For this review, take the finished solid that the model builds, in its own axes (mm). A direction names the side the tool comes from. Coordinates: 2 decimals unless noted, no trailing zeros. Write each loop counter-clockwise with the first axis right and the second up, starting at its lowest first coordinate (ties: lowest second). Pieces come first, ordered by that corner, then holes.
Autodesk Inventor part; units mm, degrees
ref_plane "YZ Plane" through (0, 0, 0) normal (1, 0, 0) x (0, 1, 0)
ref_plane "XZ Plane" through (0, 0, 0) normal (0, 1, 0) x (-1, 0, 0)
ref_plane "XY Plane" through (0, 0, 0) normal (0, 0, 1) x (1, 0, 0)
ref_plane "Plano de trabajo1" through (0, 0, 0) normal (0, 0, 1) x (1, 0, 0)
sketch "Boceto1" plane through (0, 0, 0) normal (0, 0, 1) x (1, 0, 0)
  circle A0 centre (10.9923, -7.35) radius 1.2028
  circle A1 centre (3.6423, 0) radius 1.2028
  circle A2 centre (18.3423, 0) radius 1.2028
  circle A3 centre (10.9923, 7.35) radius 1.2028
  circle A4 centre (10.9923, 0) radius 10.9823
  line L0 (10.9923, -10.9823) -> (-139.0077, -10.9823)
  line L1 (10.9923, 10.9823) -> (-139.0077, 10.9823)
  line L2 (-139.0077, 10.9823) -> (-139.0077, -10.9823)
  point P0 (0, 0)
  dimension "d0" = 150
  dimension "d1" = 150
extrude "Extrusión1" add sketch "Boceto1" along normal blind 3
sketch "Boceto2" plane through (0, 0, 3) normal (0, 0, 1) x (1, 0, 0)
  arc A0 (-129.1978, -5.6745) -> (-132.1454, -8.5217) centre (-128.1245, -9.7351) ccw
  circle A1 centre (-128.1245, 8.4649) radius 0.85 construction
  circle A2 centre (-128.1245, -9.7351) radius 0.7049 construction
  line L0 (-139.0305, -11.0697) -> (-267.2186, 10.8953)
  line L1 (-267.2186, -11.0694) -> (-117.2186, -11.0694)
  line L2 (-139.0305, 10.8953) -> (-139.0305, -11.0694)
  line L3 (-117.2186, 10.8953) -> (-267.2186, 10.8953)
  line L4 (-128.1245, -11.0697) -> (-128.1245, -0.0872)
  line L5 (-128.1245, -0.0872) -> (-128.1245, 9.0128)
  line L6 (-128.1245, -0.0872) -> (-128.1245, -9.1872)
  circle A3 centre (-128.1245, -9.1872) radius 0.85
  circle A4 centre (-128.1245, 9.0128) radius 0.85
  circle A5 centre (-128.1245, -9.1872) radius 1.8825
  circle A6 centre (-128.1245, 9.0128) radius 1.8821
  circle A7 centre (-128.1245, 9.0128) radius 0.85
  circle A8 centre (-128.1245, -9.1872) radius 0.85
  line L7 (-128.1245, 10.8953) -> (-139.0305, 10.8953)
  line L8 (-139.0077, 10.9823) -> (-139.0077, -10.9823)
  line L9 (-139.0077, -10.9823) -> (-139.0077, 10.9823)
  line L10 (-139.0077, 10.9823) -> (-139.0077, -10.9823)
  point P0 (0, 0)
  dimension "d4" = 10.9825
  dimension "d5" = 9.1
  dimension "d6" = 9.1
  dimension "d7" = 1.7
  dimension "d8" = 1.7
extrude "Extrusión2" cut sketch "Boceto2" against normal blind 3 contours A3 L4 | L4 A3 | A4
sketch "Boceto3" plane through (0, 0, 3) normal (0, 0, 1) x (1, 0, 0)
  circle A0 centre (-128.1245, -9.1872) radius 0.85
  circle A1 centre (-128.1245, 9.0128) radius 0.85
  line L0 (10.9923, 10.9823) -> (-139.0077, 10.9823)
  line L1 (-139.0077, 10.9823) -> (-139.0077, -10.9823)
  line L2 (-139.0077, -10.9823) -> (10.9923, -10.9823)
  arc A2 (10.9923, -10.9823) -> (10.9923, 10.9823) centre (10.9923, 0) ccw
  circle A3 centre (10.9923, -7.35) radius 1.2028
  circle A4 centre (3.6423, 0) radius 1.2028
  circle A5 centre (18.3423, 0) radius 1.2028
  circle A6 centre (10.9923, 7.35) radius 1.2028
  line L3 (-130.1442, 5.5225) -> (-129.5361, 14.2169)
  circle A7 centre (-128.1245, -9.1872) radius 1.7951
  circle A8 centre (-128.1245, 9.0128) radius 1.9695
  line L4 (-128.1245, -7.3921) -> (-128.1245, 7.0432)
  line L5 (-128.1245, -10.9823) -> (-128.1245, -18.0451)
  line L6 (-128.1245, -18.0451) -> (-142.6221, -18.554)
  line L7 (-142.6221, -18.554) -> (-141.7315, 12.8288)
  line L8 (-141.7315, 12.8288) -> (-128.1245, 12.4426)
  line L9 (-128.1245, 12.4426) -> (-128.1245, 10.9823)
  point P0 (0, 0)
extrude "Extrusión3" cut sketch "Boceto3" against normal blind 3 contours A8 L3 L0 | L3 A8 L4 A7 L2 L1 L0
sketch "Boceto4" plane through (0, 0, 0) normal (0, 0, -1) x (-1, 0, 0)
  arc A0 (128.1245, 7.0432) -> (128.1245, 10.9823) centre (128.1245, 9.0128) ccw
  line L0 (-10.9923, 10.9823) -> (128.1245, 10.9823)
  arc A1 (-10.9923, 10.9823) -> (-10.9923, -10.9823) centre (-10.9923, 0) ccw
  line L1 (128.1245, -10.9823) -> (-10.9923, -10.9823)
  arc A2 (128.1245, -10.9823) -> (128.1245, -7.3921) centre (128.1245, -9.1872) ccw
  line L2 (128.1245, -7.3921) -> (128.1245, 7.0432)
  circle A3 centre (128.1245, -9.1872) radius 0.85
  circle A4 centre (128.1245, 9.0128) radius 0.85
  circle A5 centre (-10.9923, -7.35) radius 1.2028
  circle A6 centre (-3.6423, 0) radius 1.2028
  circle A7 centre (-18.3423, 0) radius 1.2028
  circle A8 centre (-10.9923, 7.35) radius 1.2028
  line L3 (108.1857, 10.9823) -> (108.1857, -10.9823)
  point P0 (0, 0)
extrude "Extrusión4" add sketch "Boceto4" along normal blind 12 contours L2 A2 L1 L3 L0 A0
sketch "Boceto5" plane through (0, 0, 3) normal (0, 0, 1) x (1, 0, 0)
  line L0 (-108.1857, -10.9823) -> (-108.1857, 10.9823)
  circle A0 centre (10.9923, 7.35) radius 1.2028
  circle A1 centre (18.3423, 0) radius 1.2028
  circle A2 centre (3.6423, 0) radius 1.2028
  circle A3 centre (10.9923, -7.35) radius 1.2028
  arc A4 (-128.1245, 10.9823) -> (-128.1245, 7.0432) centre (-128.1245, 9.0128) ccw
  line L1 (-128.1245, 7.0432) -> (-128.1245, -7.3921)
  arc A5 (-128.1245, -7.3921) -> (-128.1245, -10.9823) centre (-128.1245, -9.1872) ccw
  line L2 (-128.1245, -10.9823) -> (10.9923, -10.9823)
  arc A6 (10.9923, -10.9823) -> (10.9923, 10.9823) centre (10.9923, 0) ccw
  line L3 (10.9923, 10.9823) -> (-128.1245, 10.9823)
  circle A7 centre (-128.1245, 9.0128) radius 0.85
  circle A8 centre (-128.1245, -9.1872) radius 0.85
  line L4 (-108.1857, 10.9823) -> (-111.1857, 10.9823)
  line L5 (-111.1857, 10.9823) -> (-111.1857, -10.9823)
  line L6 (-111.1857, -10.9823) -> (-108.1857, -10.9823)
  line L7 (-108.1857, -10.9823) -> (-108.1857, 10.9823)
  line L8 (10.9923, 10.9823) -> (-128.1245, 10.9823)
  line L9 (-122.3999, 10.9823) -> (-122.3999, -10.9823)
  point P0 (0, 0)
  dimension "d15" = 3
extrude "Extrusión5" cut sketch "Boceto5" against normal blind 13 contours L2 A5 L1 A4 L3 L9
chamfer "Chaflán1" distance 12 angle 45 1 edges at (-122.3999, 0, 3)
chamfer "Chaflán2" distance 12 angle 45 1 edges at (-108.1857, 0, -12)
sketch "Boceto6" plane through (0, 0, -12) normal (0, 0, -1) x (-1, 0, 0)
  line L0 (126.0445, -11.1372) -> (126.0445, 10.9228)
  line L1 (120.1857, -10.9823) -> (120.1857, 10.9823)
  line L2 (120.1857, -10.9823) -> (128.1245, -10.9823)
  line L3 (120.1857, 10.9823) -> (122.6857, 10.9823)
  line L4 (122.6857, 10.9823) -> (122.6857, -10.9823)
  line L5 (122.6857, -10.9823) -> (120.1857, -10.9823)
  line L6 (120.1857, -10.9823) -> (120.1857, 10.9823)
  point P0 (0, 0)
  dimension "d24" = 2.5
extrude "Extrusión6" add sketch "Boceto6" along normal blind 20
sketch "Boceto7" plane through (-128.1245, -10.9823, -10) normal (0, -1, 0) x (1, 0, 0)
  line L0 (19.9388, 10) -> (7.9388, -2)
  line L1 (19.9388, 10) -> (139.1168, 10)
  line L2 (139.1168, 10) -> (139.1168, 13)
  line L3 (17.7246, 13) -> (139.1168, 13)
  line L4 (5.7246, 1) -> (17.7246, 13)
  line L5 (5.7246, 1) -> (5.7246, 0)
  line L6 (5.7246, 0) -> (0, 0)
  line L7 (0, 0) -> (0, -2)
  line L8 (5.4388, -2) -> (0, -2)
  line L9 (5.4388, -2) -> (5.4388, -22)
  line L10 (7.9388, -22) -> (5.4388, -22)
  line L11 (7.9388, -2) -> (7.9388, -22)
  line L12 (7.9388, -2) -> (7.9388, -22)
  line L13 (5.4388, -22) -> (7.9388, -22)
  line L14 (7.9388, -22) -> (7.9388, -4)
  line L15 (7.9388, -4) -> (5.4388, -4)
  line L16 (5.4388, -4) -> (5.4388, -22)
  point P0 (128.1245, 10)
  point P1 (5.4388, -4)
  dimension "d27" = 18
extrude "Extrusión7" add sketch "Boceto7" along normal blind 2 contours L11 L10 L9 L15
sketch "Boceto8" plane through (-122.6857, -10.9823, -12) normal (-1, 0, 0) x (0, 0, 1)
  line L0 (0, 21.9646) -> (0, 0)
  line L1 (0, 21.9646) -> (-20, 21.9646)
  line L2 (-20, 21.9646) -> (-20, -2)
  line L3 (-2, -2) -> (-20, -2)
  line L4 (-2, 0) -> (-2, -2)
  line L5 (0, 0) -> (-2, 0)
  line L6 (-20, 0) -> (-2, 0)
  point P0 (12, 10.9823)
extrude "Extrusión8" add sketch "Boceto8" along normal blind 50 contours L4 L3 L2 L6
sketch "Boceto9" plane through (-120.1857, -12.9823, -14) normal (0, 0, 1) x (1, 0, 0)
  line L0 (-2.5, 2) -> (0, 2)
  line L1 (-2.5, 2) -> (-52.5, 2)
  line L2 (-52.5, 0) -> (-52.5, 2)
  line L3 (0, 0) -> (-52.5, 0)
  line L4 (0, 2) -> (0, 0)
  line L5 (-2.5, 0) -> (-52.5, 0)
  line L6 (-52.5, 0) -> (-52.5, 2)
  line L7 (-52.5, 2) -> (-2.5, 2)
  line L8 (-2.5, 2) -> (-2.5, 0)
  point P0 (120.1857, 12.9823)
extrude "Extrusión9" add sketch "Boceto9" along normal blind 4 contours L8 L3 L2 L1
sketch "Boceto10" plane through (0, 0, -32) normal (0, 0, -1) x (-1, 0, 0)
  line L0 (120.1857, 10.9823) -> (120.1857, -12.9823)
  line L1 (120.1857, -12.9823) -> (172.6857, -12.9823)
  line L2 (172.6857, -10.9823) -> (172.6857, -12.9823)
  line L3 (122.6857, -10.9823) -> (172.6857, -10.9823)
  line L4 (122.6857, 10.9823) -> (122.6857, -10.9823)
  line L5 (122.6857, 10.9823) -> (120.1857, 10.9823)
  line L6 (133.3495, -12.9823) -> (133.3495, -10.9823)
  line L7 (128.1245, -10.9823) -> (172.6857, -10.9823)
  point P0 (0, 0)
extrude "Extrusión10" add sketch "Boceto10" along normal blind 8 contours L6 L3 L2 L1
sketch "Boceto11" plane through (-172.6857, -10.9823, -10) normal (0, 1, 0) x (1, 0, 0)
  line L0 (50, 22) -> (50, 4)
  line L1 (50, 22) -> (39.3362, 22)
  line L2 (39.3362, 22) -> (39.3362, 30)
  line L3 (0, 30) -> (39.3362, 30)
  line L4 (0, 30) -> (0, 0)
  line L5 (44.5612, 0) -> (0, 0)
  line L6 (44.5612, 0) -> (44.5612, 2)
  line L7 (50, 2) -> (44.5612, 2)
  line L8 (50, 2) -> (50, 4)
  line L9 (39.3362, 22) -> (39.3362, 30)
  line L10 (39.3362, 30) -> (39.3362, 28)
  line L11 (39.3362, 28) -> (0, 28)
  line L12 (0, 28) -> (2, 28)
  line L13 (2, 28) -> (2, 0)
  line L14 (0, 0) -> (0, 30)
  line L15 (0, 0) -> (0, 2)
  line L16 (0, 2) -> (43.0714, 2)
  line L17 (43.0714, 2) -> (43.0714, 0)
  line L18 (44.5612, 0) -> (0, 0)
  point P0 (172.6857, -10)
  point P1 (2, 2)
  point P2 (39.3362, 28)
  dimension "d36" = 2
  dimension "d37" = 2
  dimension "d38" = 2
extrude "Extrusión11" add sketch "Boceto11" along normal blind 3 contours L11 L4 L3 L2 | L13 L16 L4 L11 | L16 L17 L5 L13 | L13 L5 L4 L16
sketch "Boceto12" plane through (0, 0, -40) normal (0, 0, -1) x (-1, 0, 0)
  circle A0 centre (168.3345, -9.2072) radius 0.85
  point P0 (0, 0)
extrude "Extrusión12" cut sketch "Boceto12" against normal blind 35
sketch "Boceto13" plane through (0, 0, -12) normal (0, 0, -1) x (-1, 0, 0)
  circle A0 centre (168.3345, -9.2072) radius 0.85
  circle A1 centre (128.1245, 9.0128) radius 0.85
  circle A2 centre (128.1245, -9.1872) radius 0.85
  arc A3 (129.6143, -8.1857) -> (128.1245, -7.3921) centre (128.1245, -9.1872) ccw
  line L0 (128.1245, -7.3921) -> (128.1245, 7.0432)
  arc A4 (128.1245, 7.0432) -> (128.1245, 10.9823) centre (128.1245, 9.0128) ccw
  line L1 (128.1245, 10.9823) -> (122.6857, 10.9823)
  line L2 (122.6857, 10.9823) -> (122.6857, -10.9823)
  line L3 (122.6857, -10.9823) -> (128.1245, -10.9823)
  arc A5 (128.1245, -10.9823) -> (129.6143, -10.1887) centre (128.1245, -9.1872) ccw
  line L4 (129.6143, -10.9823) -> (129.6143, -10.1887)
  line L5 (170.6857, -10.9823) -> (129.6143, -10.9823)
  line L6 (170.6857, -10.9823) -> (170.6857, -7.9823)
  line L7 (129.6143, -7.9823) -> (170.6857, -7.9823)
  line L8 (129.6143, -8.1857) -> (129.6143, -7.9823)
  circle A6 centre (128.1245, 9.0128) radius 2.7195
  circle A7 centre (128.1245, -9.1872) radius 2.545
  point P0 (0, 0)
  point P1 (126.3205, -10.9823)
  point P2 (129.9286, -10.9823)
  point P3 (130.3662, -7.9823)
  point P4 (128.1245, -6.6422)
  point P5 (128.1245, 6.2933)
  point P6 (126.2493, 10.9823)
  dimension "d43" = 5.439
  dimension "d44" = 5.09
extrude "Extrusión13" add sketch "Boceto13" against normal blind 2 contours A3 L0 A7 L7 L8 | L0 A4 L1 A6 | L3 A5 L4 L5 A7 picked at (127.0429, 11.109)
sketch "Boceto14" plane through (0, 0, -10) normal (0, 0, 1) x (1, 0, 0)
  circle A0 centre (-128.1245, -9.1872) radius 0.85
  arc A1 (-128.1245, -6.6422) -> (-130.3662, -7.9823) centre (-128.1245, -9.1872) ccw
  circle A2 centre (-168.3345, -9.2072) radius 0.85
  circle A3 centre (-168.3345, -9.2072) radius 0.85
  circle A4 centre (-168.3345, -9.2072) radius 2.545
  line L0 (-172.6857, -7.9823) -> (-130.3662, -7.9823)
  point P0 (0, 0)
  point P1 (-170.5654, -7.9823)
  point P2 (-166.1037, -7.9823)
  dimension "d47" = 5.09
extrude "Extrusión14" add sketch "Boceto14" against normal blind 2 contours L0 A4 picked at (-168.0387, -7.2686)
sketch "Boceto15" plane through (0, 0, -40) normal (0, 0, -1) x (-1, 0, 0)
  circle A0 centre (168.3345, -9.2072) radius 0.85
  circle A1 centre (168.3345, -9.2072) radius 2.545
  line L0 (133.3495, -7.9823) -> (172.6857, -7.9823)
  point P0 (0, 0)
  point P1 (166.1037, -7.9823)
  point P2 (170.5654, -7.9823)
  dimension "d50" = 5.09
extrude "Extrusión15" add sketch "Boceto15" against normal blind 2 contours L0 A1 picked at (168.6303, -7.2686)
properties part number "femurAux"
Q1. Tool access review of faces 4 (the flat face through (-120.186, -1, -22)), 5 (the flat face through (-152, -9, -38)), 6 (the flat face through (-146, -10.982, -25)), 7 (the flat face through (-146, -12.982, -25)), 8 (the flat face through (-45, 0, 3)): name each direction out of +Z, -Z, +X, -X, +Y, -Y from which nothing blocks a thin tool from reaching the whole face with its end or side.
Ans:
face 4: -Z, +X, +Y, -Y
face 5: +X, +Y
face 6: +Y
face 7: +Z, -Z, +X, -X, -Y
face 8: +Z, +X, -X, +Y, -Y
Q2. Add section D-D (z = -3). State the section outline as (x, y) points.
Ans:
outline: (-116.4, -10.98) - (-111.19, -10.98) - (-111.19, 10.98) - (-116.4, 10.98) - close
Q3. Draft analysis for pull direction Z (two halves, no side actions). For faces 1 (the flat face through (-153, -10, -40)), 2 (the flat face through (-140, -9, -10)), 3 (the flat face through (-138, -10, -12)), state which applies: +Z half, -Z half, draft (parallel to the pull), parting line (faces both ways), or undercut.
Ans:
face 1: -Z half
face 2: +Z half
face 3: undercut
Q4. Add section C-C (z = -34). State the section outline as (x, y) points.
Ans:
outline: (-172.69, -12.98) - (-133.35, -12.98) - (-133.35, -10.98) - (-170.69, -10.98) - (-170.69, -7.98) - (-172.69, -7.98) - close
Q5. Add section A-A (z = -18). State the section outline as (x, y) points, then the cut area to 3 significant figures.
Ans:
outline: (-172.69, -12.98) - (-120.19, -12.98) - (-120.19, 10.98) - (-122.69, 10.98) - (-122.69, -10.98) - (-170.69, -10.98) - (-170.69, -7.98) - (-172.69, -7.98) - close
area: 166 mm2
Q6. Add section B-B (x = -14.5). State the section outline as (y, z) points.
Ans:
outline: (-10.98, 0) - (10.98, 0) - (10.98, 3) - (-10.98, 3) - close
Q7. For probe 1 along Z at (x, y) = (-82, 3.25); probe 2 along X at (y, z) = (-2, -24); probe 3 along Y at (x, z) = (-128, -29.5), list the stretches that pass through material, from the lowest coordinate up.
Ans:
probe 1: z = 0 to 3
probe 2: x = -122.69 to -120.19
probe 3: y = -12.98 to -10.98
Q8. Clearance check with flat-ended pins moving along their axes: pin 1 Ø13.5 at (x, z) = (-25, -8) entering from -Y; pin 2 Ø21 at (x, z) = (-142.5, -28) entering from +Y; pin 3 Ø0.6 at (y, z) = (-1, -11) entering from -X; pin 4 Ø2.5 at (x, y) = (-128.12, 9.01) entering from -Z. State where each tip first meets the part, or that it passes through.
Ans:
pin 1: passes through
pin 2: stops at y = -7.98
pin 3: stops at x = -128.12
pin 4: stops at z = -12
